```python
from build123d import *

# Parameters (mm, degrees)
SKETCH1_W           = 19
SKETCH1_H           = 21.9
BOSS_EXTRUDE1_DEPTH = 0.82
SKETCH2_W           = 18.6
SKETCH2_H           = 19.45
BOSS_EXTRUDE2_DEPTH = 2.18
SKETCH3_R           = 0.35
CUT_EXTRUDE1_DEPTH  = 30.075116509


with BuildPart() as part:
    # Sketch1 → Boss-Extrude1 (new body)
    with BuildSketch(Plane.XY):
        with Locations((9.5, 10.95)):
            Rectangle(SKETCH1_W, SKETCH1_H)
    extrude(amount=BOSS_EXTRUDE1_DEPTH)

    # Sketch2 → Boss-Extrude2 (add)
    with BuildSketch(Plane.XY.offset(0.82)):
        with Locations((9.5, 10.95)):
            Rectangle(SKETCH2_W, SKETCH2_H)
    extrude(amount=BOSS_EXTRUDE2_DEPTH)

    # Sketch3 → Cut-Extrude1 (cut, through all)
    with BuildSketch(Plane.XY.offset(0.82)):
        with Locations((4.5, 21.9)):
            Circle(SKETCH3_R)
        with Locations((7, 21.9)):
            Circle(SKETCH3_R)
        with Locations((9.5, 21.9)):
            Circle(SKETCH3_R)
        with Locations((12, 21.9)):
            Circle(SKETCH3_R)
        with Locations((14.5, 21.9)):
            Circle(SKETCH3_R)
        with Locations((4.3, 0)):
            Circle(SKETCH3_R)
        with Locations((6.9, 0)):
            Circle(SKETCH3_R)
        with Locations((9.5, 0)):
            Circle(SKETCH3_R)
        with Locations((12.1, 0)):
            Circle(SKETCH3_R)
        with Locations((14.7, 0)):
            Circle(SKETCH3_R)
        with Locations((17.3, 0)):
            Circle(SKETCH3_R)
    extrude(amount=-CUT_EXTRUDE1_DEPTH, mode=Mode.SUBTRACT)


solid = part.part
```
Read the model definition and answer for the solid it produces. Units are mm, in the model's axes. A direction names the side the tool comes from. Round coordinates to 2 decimals unless told otherwise and drop trailing zeros. Loops run counter-clockwise (first coordinate to the right, second up) from the corner with the lowest first, then second, coordinate; pieces in that order, holes last. Notation, with made-up numbers: (8.25, -13) -> (62.25, -13) arc R21 cw to (62.25, 0) -> close; hole circle Ø2 at (0.25, 20). An arc over 180 degrees is marked (long way). One line per item, written item: value.
1) A cutting plane is placed at C-C (z = 2.3). Determine the outline of the cut face in (x, y) (3 decimals).
Answer list:
outline: (0.2, 1.225) -> (18.8, 1.225) -> (18.8, 20.675) -> (0.2, 20.675) -> close
2) Flat-ended cylindrical pins translate along their axes: P1, Ø0.7, axis at x = 12, z = 2, coming from the +Y side (3 decimals); P2, Ø1, axis at y = 16, z = 1.5, coming from the +X side. Find the tip coordinate at first contact, or state that the pin passes through.
Answer list:
P1: stops at y = 20.675
P2: stops at x = 18.8
3) A cutting plane is placed at A-A (x = 17.3). Determine the outline of the cut face in (y, z) (3 decimals), and give its area (3 significant figures).
Answer list:
outline: (0.35, 0) -> (21.9, 0) -> (21.9, 0.82) -> (20.675, 0.82) -> (20.675, 3) -> (1.225, 3) -> (1.225, 0.82) -> (0.35, 0.82) -> close
area: 60.1 mm²
4) A cutting plane is placed at B-B (y = 6.25). Determine the outline of the cut face in (x, z).
Answer list:
outline: (0, 0) -> (19, 0) -> (19, 0.82) -> (18.8, 0.82) -> (18.8, 3) -> (0.2, 3) -> (0.2, 0.82) -> (0, 0.82) -> close
5) Consider L1, parallel to X at y = 14.75, z = 1.9; L2, parallel to Y at x = 9, z = 1.1 (3 decimals). Determine where each line is inside the solid, lowest interval first. Write a range as [from, to].
Answer list:
L1: x = [0.2, 18.8]
L2: y = [1.225, 20.675]
6) For faces 1 (the face through (18.8, 11, 2)), 2 (the face through (0.2, 11, 2)), 3 (the face through (9, 20.675, 2)), determine the directions among +Z, -Z, +X, -X, +Y, -Y from which every point of the face is accessible in a straight line to the end or side of a thin tool.
Answer list:
face 1: +Z, +X, +Y, -Y
face 2: +Z, -X, +Y, -Y
face 3: +Z, +X, -X, +Y
7) The mould has two halves that part along Z. Classify faces 4 (the face through (18.3, 0, 0.4)), 5 (the face through (9, 11, 0)), 6 (the face through (9, 11, 3)): pulls with the +Z half, pulls with the -Z half, needs draft (parallel to the pull), parting line crosses it, or undercut.
Answer list:
face 4: needs draft
face 5: pulls with the -Z half
face 6: pulls with the +Z half
